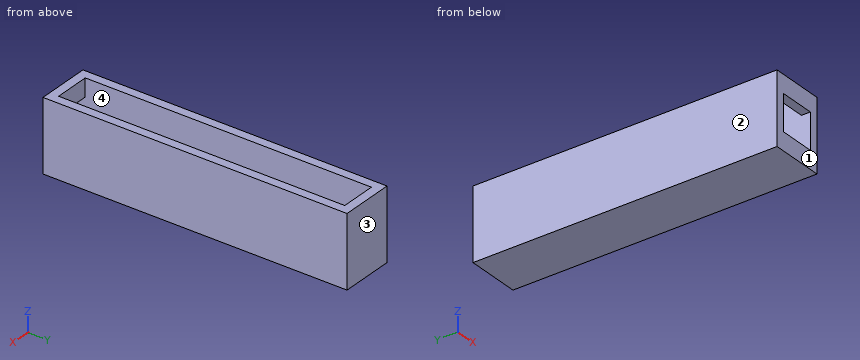
```python
from build123d import *

# Parameters (mm, degrees)
F0_W     = 19.05
F0_H     = 107.95
F0_W_2   = 12.7
F0_H_2   = 101.6
F1_DEPTH = 25.4
F2_DEPTH = 6.35
F3_W     = 12.7
F3_H     = 12.7
F4_DEPTH = 25.4


with BuildPart() as f1:
    # F0 (on Top) → F1 (new body)
    with BuildSketch(Plane.XY):
        with Locations((-21.172236, -17.613889)):
            Rectangle(F0_W, F0_H)
        with Locations((-21.172236, -17.613889)):
            Rectangle(F0_W_2, F0_H_2, mode=Mode.SUBTRACT)
    extrude(amount=F1_DEPTH)

    # F0 (on Top) → F2 (join)
    with BuildSketch(Plane.XY):
        with Locations((-21.172236, -17.613889)):
            Rectangle(F0_W_2, F0_H_2)
    extrude(amount=F2_DEPTH)

    # F3 (on face) → F4 (cut)
    with BuildSketch(Plane.XZ.offset(71.588889)):
        with Locations((-21.172236, 12.7)):
            Rectangle(F3_W, F3_H)
    extrude(amount=-F4_DEPTH, mode=Mode.SUBTRACT)


solid = f1.part
```
The listing builds one solid part. Answer for the finished solid, in the listing's coordinates (mm). Face numbers are marked on the shaded views. Coordinates: 2 decimals unless noted, no trailing zeros. Write each loop counter-clockwise with the first axis right and the second up, starting at its lowest first coordinate (ties: lowest second). Pieces come first, ordered by that corner, then holes.
Q1. Section A-A, the plane x = -15.75 is taken. Write down the section's boundary in (y, z).
Returned:
outline: (-71.59, 0) - (36.36, 0) - (36.36, 25.4) - (33.19, 25.4) - (33.19, 6.35) - (-71.59, 6.35) - close; (-71.59, 19.05) - (-68.41, 19.05) - (-68.41, 25.4) - (-71.59, 25.4) - close
Q2. Section B-B, the plane z = 8.5 is taken. Write down the section's boundary in (x, y), then the cut area to 3 significant figures.
Returned:
outline: (-30.7, -71.59) - (-27.52, -71.59) - (-27.52, 33.19) - (-14.82, 33.19) - (-14.82, -71.59) - (-11.65, -71.59) - (-11.65, 36.36) - (-30.7, 36.36) - close
area: 726 mm2
Q3. The mould has two halves that part along Y. Classify the marked faces 1, 2, 3 and 4: released by +Y, released by -Y, zero draft, split by the parting line, or undercut.
Returned:
face 1: released by -Y
face 2: zero draft
face 3: released by +Y
face 4: undercut
Q4. Section C-C, the plane y = 3 is taken. Write down the section's boundary in (x, z).
Returned:
outline: (-30.7, 0) - (-11.65, 0) - (-11.65, 25.4) - (-14.82, 25.4) - (-14.82, 6.35) - (-27.52, 6.35) - (-27.52, 25.4) - (-30.7, 25.4) - close
Q5. Given P1, Ø5, axis at x = -21.5, y = -43.5, coming from the +Z side; P2, Ø4, axis at x = -23, z = 12.5, coming from the -Y side, each flat-ended and moving along its own axis, determine where each tip first touches the part or whether it passes through.
Returned:
P1: stops at z = 6.35
P2: stops at y = 33.19
Q6. Find the intervals of material crossed by line 1 along X through (y, z) = (21.5, 18); line 2 along Y through (x, z) = (-21, 21.75); line 3 along Z through (x, y) = (-24.25, 0.5), in increasing order.
Returned:
line 1: x = -30.7 to -27.52, -14.82 to -11.65
line 2: y = -71.59 to -68.41, 33.19 to 36.36
line 3: z = 0 to 6.35
